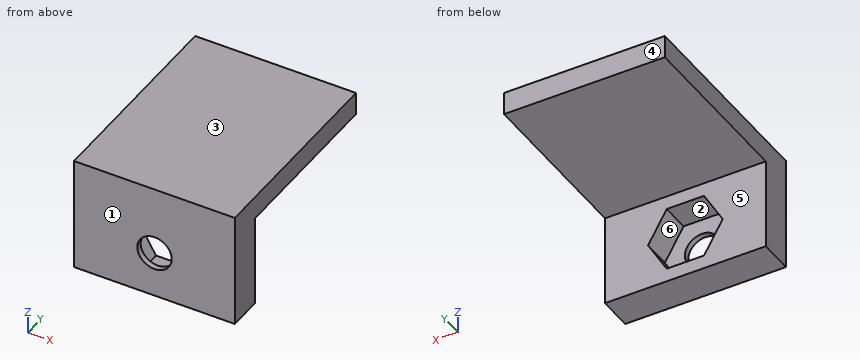
Autodesk Inventor part; units mm, degrees
ref_plane "YZ Plane" through (0, 0, 0) normal (1, 0, 0) x (0, 1, 0)
ref_plane "XZ Plane" through (0, 0, 0) normal (0, 1, 0) x (-1, 0, 0)
ref_plane "XY Plane" through (0, 0, 0) normal (0, 0, 1) x (1, 0, 0)
sketch "Sketch1" plane through (0, 0, 0) normal (0, 1, 0) x (-1, 0, 0)
  line L0 (9.8, 0) -> (-9.8, 0)
  line L1 (0, -7) -> (0, 7)
  line L2 (-7, 5) -> (7, 5)
  line L3 (7, 5) -> (7, -5)
  line L4 (7, -5) -> (-7, -5)
  line L5 (-7, -5) -> (-7, 5)
  line L6 (-7, 5) -> (7, -5) construction
  line L7 (7, 5) -> (-7, -5) construction
  point P0 (0, 0)
  dimension "d0" = 14
  dimension "d1" = 10
extrude "Extrusion1" add sketch "Sketch1" along normal blind 3
sketch "Sketch2" plane through (0, 3, 0) normal (0, 1, 0) x (1, 0, 0)
  line L0 (-7, 5) -> (-7, -5)
  line L1 (7, -5) -> (7, 5)
  line L2 (-7, -5) -> (7, -5)
  line L3 (7, -5) -> (7, -3)
  line L4 (7, -3) -> (-7, -3)
  line L5 (-7, -3) -> (-7, -5)
  point P0 (0, 0)
  point P1 (7, -5)
  point P2 (-7, -3)
  dimension "d4" = 2
extrude "Extrusion2" add sketch "Sketch2" along normal blind 15
sketch "Sketch4" plane through (0, 3, 0) normal (0, 1, 0) x (1, 0, 0)
  line L0 (1.625, -1.8146) -> (-1.625, -1.8146)
  line L1 (-1.625, -1.8146) -> (-3.25, 1)
  line L2 (-3.25, 1) -> (-1.625, 3.8146)
  line L3 (-1.625, 3.8146) -> (1.625, 3.8146)
  line L4 (1.625, 3.8146) -> (3.25, 1)
  line L5 (3.25, 1) -> (1.625, -1.8146)
  line L6 (7, 5) -> (-7, 5)
  line L7 (-7, 5) -> (-7, -3)
  point P0 (0, 0)
  point P1 (0, 1)
  dimension "d8" = 6.5
  dimension "d9" = 3.25
  dimension "d10" = 4
  dimension "d11" = 7
extrude "Extrusion3" cut sketch "Sketch4" against normal blind 2.5
sketch "Sketch5" plane through (0, 0.5, 0) normal (0, 1, 0) x (1, 0, 0)
  line L0 (-3.25, 1) -> (-1.625, 3.8146)
  line L1 (-1.625, 3.8146) -> (1.625, 3.8146)
  point P0 (0, 0)
  point P1 (0.008, 1.0001)
  dimension "d21" = 2.8215
  dimension "d22" = 2.8145
hole "Hole1" at (0.008, 0.5, -1.0001) direction (0, -1, 0) diameter 3 end through all
properties part number "uchwyt_krancowka_alternatywa_2"
Design review of the part built by this model. Coordinates are the model's own, in mm. Face numbers are marked on the shaded views. A direction names the side the tool comes from. Round coordinates to 2 decimals unless told otherwise and drop trailing zeros. Write each loop counter-clockwise with the first axis right and the second up, starting at its lowest first coordinate (ties: lowest second). Pieces come first, ordered by that corner, then holes. Notation, with made-up numbers: (49.25, 41.5) -> (60.25, 41.5) arc R27 ccw to (60.25, 73.5) -> close; hole circle Ø4 at (39.5, 13). An arc over 180 degrees is marked (long way). Answer in a Markdown table with one row per item.
Q1. Take a section at C-C, the plane x = 4. State the section outline as (y, z) points.
The answers:
| item | result |
|---|---|
| outline | (0, -5) -> (3, -5) -> (3, 3) -> (18, 3) -> (18, 5) -> (0, 5) -> close |
Q2. Take a section at B-B, the plane z = -0.25. State the section outline as (x, y) points, then the cut area to 3 significant figures.
The answers:
| item | result |
|---|---|
| outline | (-7, 0) -> (-1.29, 0) -> (-1.29, 0.5) -> (-2.82, 0.5) -> (-2.82, 3) -> (-7, 3) -> close; (1.31, 0) -> (7, 0) -> (7, 3) -> (2.82, 3) -> (2.82, 0.5) -> (1.31, 0.5) -> close |
| area | 26.6 mm² |
Q3. For the marked faces 4, 5 and 6, list the 3-axis set-ups (+Z, -Z, +X, -X, +Y, -Y) from which the entire face can be reached by the end or side of a thin tool; tool diameter is ignored.
The answers:
| item | result |
|---|---|
| face 4 | +Z, -Z, +X, -X, +Y |
| face 5 | -Z, +X, -X, +Y |
| face 6 | +Y |
Q4. Take a section at A-A, the plane x = -0.25. State the section outline as (y, z) points, then the cut area to 3 significant figures.
The answers:
| item | result |
|---|---|
| outline | (0, -5) -> (3, -5) -> (3, -3.81) -> (0.5, -3.81) -> (0.5, -2.48) -> (0, -2.48) -> close; (0, 0.48) -> (0.5, 0.48) -> (0.5, 1.81) -> (3, 1.81) -> (3, 3) -> (18, 3) -> (18, 5) -> (0, 5) -> close |
| area | 44.4 mm² |
Q5. Clearance check with flat-ended pins moving along their axes: pin 1 Ø2.5 at (x, z) = (0.01, -1) entering from +Y; pin 2 Ø4.5 at (x, z) = (0.5, -1) entering from +Y; pin 3 Ø2 at (x, y) = (-1.5, 14) entering from -Z. State where each tip first meets the part, or that it passes through.
The answers:
| item | result |
|---|---|
| pin 1 | through |
| pin 2 | y = 0.5 |
| pin 3 | z = 3 |
Q6. To check wall thickness, follow L1, parallel to Z at x = 1, y = 2.25; L2, parallel to Y at x = 4.5, z = -0.75; L3, parallel to Z at x = 2, y = 16. State the ranges of each line that lie inside material, in increasing order. Write a range as [from, to].
The answers:
| item | result |
|---|---|
| L1 | [-5, -3.81], [1.81, 5] |
| L2 | [0, 3] |
| L3 | [3, 5] |
Q7. Take a section at D-D, the plane z = 1.25. State the section outline as (x, y) points, then the cut area to 3 significant figures.
The answers:
| item | result |
|---|---|
| outline | (-7, 0) -> (7, 0) -> (7, 3) -> (1.95, 3) -> (1.95, 0.5) -> (-1.95, 0.5) -> (-1.95, 3) -> (-7, 3) -> close |
| area | 32.2 mm² |
Q8. Draft analysis for pull direction Z (two halves, no side actions). For the marked faces 1, 2 and 3, state which applies: +Z half, -Z half, draft (parallel to the pull), parting line (faces both ways), or undercut.
The answers:
| item | result |
|---|---|
| face 1 | draft |
| face 2 | undercut |
| face 3 | +Z half |
